Autodesk Fusion 360 part; units mm, degrees
sketch "Szkic1" plane through (0, 0, 0) normal (0, 0, 1) x (1, 0, 0)
  line L0 (-20, 25) -> (-20, -25)
  line L1 (-20, -25) -> (0, -25)
  line L2 (0, -25) -> (0, 25)
  line L3 (0, 25) -> (-20, 25)
  line L4 (0, 10) -> (0, -10)
  line L5 (0, -10) -> (20, -10)
  line L6 (20, -10) -> (20, 10)
  line L7 (20, 10) -> (0, 10)
  circle A0 centre (10, 0) radius 3
  circle A1 centre (10, 0) radius 5.5
  line L8 (-12.5, 25) -> (-7.5, 25)
  line L9 (-7.5, 25) -> (-7.5, -25)
  line L10 (-7.5, -25) -> (-12.5, -25)
  line L11 (-12.5, -25) -> (-12.5, 25)
  dimension "d1" = 6
  dimension "d2" = 11
extrude "Wyciągnięcie proste1" add sketch "Szkic1" against normal blind 25 contours L0 L1 L3 L11 | L1 L3 L8 L9 L10 L11 | L1 L2 L3 L4 L9 | L2 L4 L5 L6 L7
extrude "Wyciągnięcie proste2" add sketch "Szkic1" against normal blind 4.2 contours A0 | A1
extrude "Wyciągnięcie proste3" cut sketch "Szkic1" against normal blind 4 contours A0
extrude "Wyciągnięcie proste4" add sketch "Szkic1" along normal blind 5 contours L1 L3 L8 L9 L10 L11
chamfer "Fazowanie1" distance 5 angle 45 1 edges at (0, -10, -12.5)
chamfer "Fazowanie2" distance 5 angle 45 1 edges at (0, 10, -12.5)
chamfer "Fazowanie3" distance 3 angle 45 6 edges at (20, 10, -12.5) (20, -10, -12.5) (0, 25, -12.5) (-20, 25, -12.5) (-20, -25, -12.5) (0, -25, -12.5)
chamfer "Fazowanie4" distance 1 angle 45 1 faces at (-11.8333, 0, -25)
delete_face "Usuń powierzchnię1" 1 faces at (16.159, -0.3074, -24.6667)
sketch "Szkic2" plane through (-20, 0, 0) normal (-1, 0, 0) x (0, -1, 0)
  line L0 (-22, -24) -> (22, -24)
  line L1 (22, -24) -> (22, 0)
  line L2 (22, 0) -> (-22, 0)
  line L3 (-22, 0) -> (-22, -24)
  line L4 (0, -12) -> (12.5, -12)
  line L5 (0, -12) -> (-12.5, -12)
  line L6 (0, -12) -> (12.5, -12)
  line L7 (0, -12) -> (-12.5, -12)
  line L8 (17.5, -4.5) -> (-17.5, -4.5)
  line L9 (-17.5, -4.5) -> (-17.5, -19.5)
  line L10 (-17.5, -19.5) -> (17.5, -19.5)
  line L11 (17.5, -19.5) -> (17.5, -4.5)
  line L12 (17.5, -4.5) -> (-17.5, -19.5) construction
  line L13 (-17.5, -4.5) -> (17.5, -19.5) construction
  line L14 (11, -5.5) -> (-11, -5.5)
  line L15 (-11, -5.5) -> (-11, -18.5)
  line L16 (-11, -18.5) -> (11, -18.5)
  line L17 (11, -18.5) -> (11, -5.5)
  line L18 (11, -5.5) -> (-11, -18.5) construction
  line L19 (-11, -5.5) -> (11, -18.5) construction
  circle A0 centre (-14.25, -12) radius 2
  circle A1 centre (14.25, -12) radius 2
  line L20 (6, -16) -> (-6, -16)
  line L21 (-6, -16) -> (-6, -8)
  line L22 (-6, -8) -> (6, -8)
  line L23 (6, -8) -> (6, -16)
  line L24 (6, -16) -> (-6, -8) construction
  line L25 (-6, -16) -> (6, -8) construction
  point P0 (0, -12)
  point P1 (0, -12)
  point P2 (0, -12)
  dimension "d15" = 12.5
  dimension "d16" = 12.5
  dimension "d18" = 4
  dimension "d19" = 4
extrude "Wyciągnięcie proste5" cut sketch "Szkic2" against normal blind 15 contours L4 L5 L6 L7 L21 L22 L23 | L4 L5 L6 L7 L20 L21 L23 | L4 L5 L6 L7 L14 L15 L17 L21 L22 L23 | L4 L5 L6 L7 L15 L16 L17 L20 L21 L23
extrude "Wyciągnięcie proste6" cut sketch "Szkic2" against normal blind 300 contours L4 L5 L6 L7 L21 L22 L23 | L4 L5 L6 L7 L20 L21 L23
extrude "Wyciągnięcie proste7" cut sketch "Szkic2" against normal blind 15 contours A1 | A0
sketch "Szkic3" plane through (0, 0, -8) normal (0, 0, -1) x (1, 0, 0)
  line L0 (-5, 6) -> (-5, -6)
  line L1 (-5, -6) -> (20, -6)
  line L2 (20, -6) -> (20, 6)
  line L3 (20, 6) -> (-5, 6)
  circle A0 centre (10, 0) radius 5.5
extrude "Wyciągnięcie proste8" add sketch "Szkic3" along normal blind 0.2 contours L0 L1 L2 L3 | A0
The listing builds one solid part. Answer for the finished solid, in the listing's coordinates (mm). A direction names the side the tool comes from. Give positions to 0.01 mm unless a question says otherwise; leave off trailing zeros. Order: outer loops, then holes, each group sorted by start corner. A loop starts at its lowest first (then second) coordinate and runs counter-clockwise, first axis right, second up. Notation, with made-up numbers: (87.5, -16) -> (132.5, -16) arc R24 cw to (132.5, 12) -> close; hole circle Ø8 at (70, 52). An arc over 180 degrees is marked (long way). Answer as a JSON object with one key per item and string values. Group by question number.
Item 1: The part is cut by section B-B on y = 0. Give the number of separate pieces and of enclosed holes in the cut face, and give its area (3 significant figures).
Item 2: Flat-ended cylindrical pins translate along their axes: pin 1 (9.5 mm diameter, centred on x = 12.5, z = -9.5, fed in from +Y); pin 2 (8 mm diameter, centred on y = -17, z = -21.5, fed in from +X); pin 3 (5.5 mm diameter, centred on x = 10, y = 0, fed in from -Z). Find the tip coordinate at first contact, or state that the pin passes through.
Item 3: Consider L1, parallel to Y at x = -9, z = -9; L2, parallel to Z at x = 17, y = 5; L3, parallel to Z at x = 7.5, y = 1.5. Determine where each line is inside the solid, lowest interval first. Write a range as from..to.
Item 4: The part is cut by section D-D on x = 10. Write down the section's boundary in (y, z).
Item 5: The part is cut by section A-A on z = -21.5. Write down the section's boundary in (x, y).
Item 6: A tool of negligible diameter and unlimited length cuts with its end or side. For faces 1 (the cylindrical face through (15.08, -2.11, -6.07)), 2 (the flat face through (-13, 11, -12)), 3 (the flat face through (7, -6, -12)), 4 (the flat face through (3, 0, 0)), 5 (the flat face through (0, 18, -12)), from which of +Z, -Z, +X, -X, +Y, -Y can it reach the whole face along a straight path? Write none if from no direction.
Item 7: The part is cut by section C-C on x = -16. Write down the section's boundary in (y, z), and give its area (3 significant figures).
Item 8: Determine the mould class of faces 6 (the cylindrical face through (12.77, -1.15, -1.97)), 7 (the flat face through (7, 6, -12)), 8 (the flat face through (2.18, 12.1, -24.51)) for opening direction Z: pulls with the +Z half, pulls with the -Z half, needs draft (parallel to the pull), parting line crosses it, or undercut.
Result set:
{
 "1": {"separate pieces": "3", "enclosed holes": "1", "area": "469 mm²"},
 "2": {"pin 1": "y = 10", "pin 2": "x = 2", "pin 3": "z = -8.2"},
 "3": {"L1": "-25..-11, 11..25", "L2": "-25..-16, -8.2..0", "L3": "-8.2..-8, -4.2..-4"},
 "4": {"outline": "(-10, -24) -> (-9, -25) -> (-5.5, -25) -> (-5.5, -16) -> (-6, -16) -> (-6, -8.2) -> (6, -8.2) -> (6, -16) -> (5.5, -16) -> (5.5, -25) -> (9, -25) -> (10, -24) -> (10, 0) -> (3, 0) -> (3, -4) -> (-3, -4) -> (-3, 0) -> (-10, 0) -> close; hole (-5.5, -8) -> (5.5, -8) -> (5.5, -4.2) -> (-5.5, -4.2) -> close"},
 "5": {"outline": "(-20, -22) -> (-17, -25) -> (-3, -25) -> (0, -22) -> (0, -15) -> (5, -10) -> (17, -10) -> (20, -7) -> (20, 7) -> (17, 10) -> (5, 10) -> (0, 15) -> (0, 22) -> (-3, 25) -> (-17, 25) -> (-20, 22) -> close; hole circle Ø11 at (10, 0)"},
 "6": {"face 1": "none", "face 2": "-X", "face 3": "+X, -X", "face 4": "+Z, +X, +Y, -Y", "face 5": "+Z, -Z, +X, +Y"},
 "7": {"outline": "(-25, -24) -> (-24, -25) -> (24, -25) -> (25, -24) -> (25, 0) -> (-25, 0) -> close; hole circle Ø4 at (-14.25, -12); hole (-11, -18.5) -> (11, -18.5) -> (11, -5.5) -> (-11, -5.5) -> close; hole circle Ø4 at (14.25, -12)", "area": "938 mm²"},
 "8": {"face 6": "needs draft", "face 7": "undercut", "face 8": "pulls with the -Z half"}
}
